CAD build for the part. Positions are in the model's coordinates, mm. Face numbers are marked on the shaded views. A direction names the side the tool comes from. Give positions to 0.01 mm unless a question says otherwise; leave off trailing zeros. Order: outer loops, then holes, each group sorted by start corner. A loop starts at its lowest first (then second) coordinate and runs counter-clockwise, first axis right, second up. Notation, with made-up numbers: (59, 7.25) -> (72, 7.25) arc R23 ccw to (72, 44.25) -> close; hole circle Ø9 at (13.25, -7.5). An arc over 180 degrees is marked (long way). Use one line per item in the form item = value. Start each with the question number.
1) Drop flat-ended pins along their axis: P1, Ø6.5, axis at x = 5, y = 18.5, coming from the +Z side; P2, Ø5.5, axis at x = 5, y = 3.56, coming from the +Z side; P3, Ø5, axis at x = 12.5, y = 23, coming from the +Z side. Give the stop position or say it passes through.
2) Probe line 1 (Y direction, x = 20, z = 0.7); line 2 (Y direction, x = 20, z = 2.7); line 3 (X direction, y = 28.5, z = 10.5). List the from-to ranges inside material, lowest first.
3) Tool access for the marked faces 1, 2 and 3: list every direction of +Z, -Z, +X, -X, +Y, -Y with a clear straight run to the whole face (end or side of a thin tool).
4) Mould opens along X. For the marked faces 4, 5, 6 and 7 say: pulls with the +X half, pulls with the -X half, needs draft (parallel to the pull), parting line crosses it, or undercut.
5) Cut at D-D, the plane y = 29. Give the cut face in (x, z).
6) Cut at B-B, the plane z = 5.75. Give the cut face in (x, y).
7) Cut at C-C, the plane x = 12.5. Give the cut face in (y, z).
8) Cut at A-A, the plane z = 15.5. Give the cut face in (x, y).
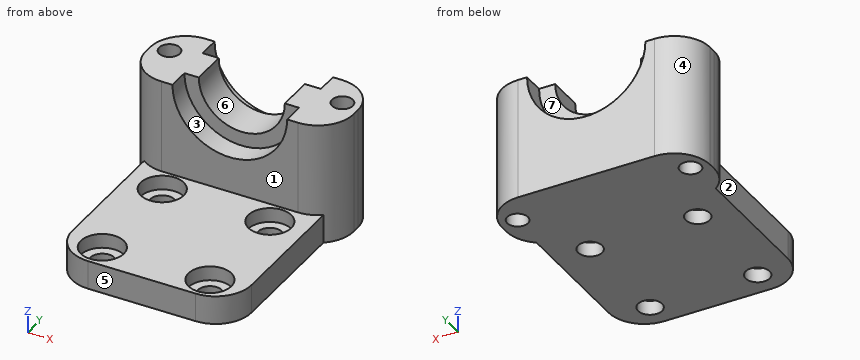
from build123d import *

# Parameters (mm, degrees)
F0_W      = 25
F0_H      = 33
F1_DEPTH  = 4
F2_R      = 1.675
F3_DEPTH  = 25
F4_W      = 25
F4_H      = 11
F5_DEPTH  = 13
F7_DEPTH  = 9
F8_R      = 8
F9_DEPTH  = 3
F2_R_2    = 3
F10_DEPTH = 2
F11_R     = 5
F12_W     = 11
F12_H     = 17
F13_DEPTH = 2
F14_W     = 11
F14_H     = 17
F15_DEPTH = 2
F16_R     = 1.45
F17_DEPTH = 25
F18_R     = 5
F19_R     = 8.25
F20_DEPTH = 3


with BuildPart() as f1:
    # F0 (on Top) → F1 (new body)
    with BuildSketch(Plane.XY):
        with Locations((12.5, 16.5)):
            Rectangle(F0_W, F0_H)
    extrude(amount=F1_DEPTH)

    # F2 (on face) → F3 (cut)
    with BuildSketch(Plane.XY.offset(4)):
        with BuildLine():
            ThreePointArc((3.325, 18.5605346784), (5, 16.8855346784), (6.675, 18.5605346784))
            ThreePointArc((6.675, 18.5605346784), (5, 20.2355346784), (3.325, 18.5605346784))
        make_face()
        with Locations((20, 18.5605346784)):
            Circle(F2_R)
        with Locations((20, 3.5605346784)):
            Circle(F2_R)
        with Locations((5, 3.5605346784)):
            Circle(F2_R)
    extrude(amount=-F3_DEPTH, mode=Mode.SUBTRACT)

    # F4 (on face) → F5 (join)
    with BuildSketch(Plane.XY.offset(4)):
        with Locations((12.5, 27.5)):
            Rectangle(F4_W, F4_H)
    extrude(amount=F5_DEPTH)

    # F6 (on face) → F7 (cut)
    with BuildSketch(Plane(origin=(0, 33, 0), x_dir=(-1, 0, 0), z_dir=(0, 1, 0))):
        with BuildLine():
            ThreePointArc((-18.5, 17), (-12.5, 11), (-6.5, 17))
            Line((-6.5, 17), (-18.5, 17))
        make_face()
    extrude(amount=-F7_DEPTH, mode=Mode.SUBTRACT)

    # F8 (on face) → F9 (cut)
    with BuildSketch(Plane.XZ.offset(-22)):
        with Locations((12.5, 17)):
            Circle(F8_R)
    extrude(amount=-F9_DEPTH, mode=Mode.SUBTRACT)

    # F2 (on face) → F10 (cut)
    with BuildSketch(Plane.XY.offset(4)):
        with BuildLine():
            ThreePointArc((8, 18.5605346784), (5, 21.5605346784), (2, 18.5605346784))
            ThreePointArc((2, 18.5605346784), (5, 15.5605346784), (8, 18.5605346784))
        make_face()
        with BuildLine():
            ThreePointArc((3.325, 18.5605346784), (5, 20.2355346784), (6.675, 18.5605346784))
            ThreePointArc((6.675, 18.5605346784), (5, 16.8855346784), (3.325, 18.5605346784))
        make_face(mode=Mode.SUBTRACT)
        with Locations((20, 18.5605346784)):
            Circle(F2_R_2)
        with Locations((20, 18.5605346784)):
            Circle(F2_R, mode=Mode.SUBTRACT)
        with Locations((20, 3.5605346784)):
            Circle(F2_R_2)
        with Locations((20, 3.5605346784)):
            Circle(F2_R, mode=Mode.SUBTRACT)
        with Locations((5, 3.5605346784)):
            Circle(F2_R_2)
        with Locations((5, 3.5605346784)):
            Circle(F2_R, mode=Mode.SUBTRACT)
    extrude(amount=-F10_DEPTH, mode=Mode.SUBTRACT)

    # F11
    f11_edges = [f1.edges().sort_by_distance(p)[0] for p in [
        (0, 0, 2),
        (25, 0, 2),
    ]]
    fillet(f11_edges, radius=F11_R)

    # F12 (on face) → F13 (join)
    with BuildSketch(Plane(origin=(0, 0, 0), x_dir=(0, -1, 0), z_dir=(-1, 0, 0))):
        with Locations((-27.5, 8.5)):
            Rectangle(F12_W, F12_H)
    extrude(amount=F13_DEPTH)

    # F14 (on face) → F15 (join)
    with BuildSketch(Plane.YZ.offset(25)):
        with Locations((27.5, 8.5)):
            Rectangle(F14_W, F14_H)
    extrude(amount=F15_DEPTH)

    # F16 (on face) → F17 (cut)
    with BuildSketch(Plane.XY.offset(17)):
        with Locations((0.45, 28.55)):
            Circle(F16_R)
        with Locations((24.55, 28.55)):
            Circle(F16_R)
    extrude(amount=-F17_DEPTH, mode=Mode.SUBTRACT)

    # F18
    f18_edges = [f1.edges().sort_by_distance(p)[0] for p in [
        (-2, 22, 8.5),
        (-2, 33, 8.5),
        (27, 33, 8.5),
        (27, 22, 8.5),
    ]]
    fillet(f18_edges, radius=F18_R)

    # F19 (on face) → F20 (cut)
    with BuildSketch(Plane(origin=(0, 33, 0), x_dir=(-1, 0, 0), z_dir=(0, 1, 0))):
        with Locations((-12.5, 17)):
            Circle(F19_R)
    extrude(amount=-F20_DEPTH, mode=Mode.SUBTRACT)


solid = f1.part
Result:
q1.P1 = 4
q1.P2 = 2
q1.P3 = 11.19
q2.line_1 = 0 to 1.89, 5.24 to 16.89, 20.24 to 33
q2.line_2 = 0 to 0.56, 6.56 to 15.56, 21.56 to 33
q2.line_3 = -1.97 to -1, 1.9 to 23.1, 26 to 26.97
q3.face_1 = +Z, +X, -X, -Y
q3.face_2 = +Z, -Z, -X, -Y
q3.face_3 = +Z, -Y
q4.face_4 = pulls with the -X half
q4.face_5 = needs draft
q4.face_6 = undercut
q4.face_7 = undercut
q5.outline = (-1.9, 0) -> (-0.93, 0) -> (-0.93, 17) -> (-1.9, 17) -> close; (1.83, 0) -> (23.17, 0) -> (23.17, 17) -> (18.5, 17) arc R6 cw to (6.5, 17) -> (1.83, 17) -> close; (25.93, 0) -> (26.9, 0) -> (26.9, 17) -> (25.93, 17) -> close
q6.outline = (-2, 27) arc R5 ccw to (3, 22) -> (22, 22) arc R5 ccw to (27, 27) -> (27, 28) arc R5 ccw to (22, 33) -> (3, 33) arc R5 ccw to (-2, 28) -> close; hole circle Ø2.9 at (0.45, 28.55); hole circle Ø2.9 at (24.55, 28.55)
q7.outline = (0, 0) -> (33, 0) -> (33, 8.75) -> (30, 8.75) -> (30, 11) -> (25, 11) -> (25, 9) -> (22, 9) -> (22, 4) -> (0, 4) -> close
q8.outline = (-2, 27) arc R5 ccw to (3, 22) -> (4.64, 22) -> (4.64, 25) -> (6.69, 25) -> (6.69, 30) -> (4.39, 30) -> (4.39, 33) -> (3, 33) arc R5 ccw to (-2, 28) -> close; (18.31, 25) -> (20.36, 25) -> (20.36, 22) -> (22, 22) arc R5 ccw to (27, 27) -> (27, 28) arc R5 ccw to (22, 33) -> (20.61, 33) -> (20.61, 30) -> (18.31, 30) -> close; hole circle Ø2.9 at (0.45, 28.55); hole circle Ø2.9 at (24.55, 28.55)
